```python
from build123d import *

# Parameters (mm, degrees)
SKETCH1_W           = 16
SKETCH1_H           = 16
BOSS_EXTRUDE1_DEPTH = 10
SKETCH4_R           = 1.75
CUT_EXTRUDE3_DEPTH  = 10
CUT_EXTRUDE4_DEPTH  = 7.5
FILLET1_R           = 1
FILLET2_R           = 1.75
FILLET5_R           = 3
CHAMFER1_SIZE       = 1
FILLET6_R           = 0.5
SKETCH6_R           = 2
CUT_EXTRUDE5_DEPTH  = 2


with BuildPart() as part:
    # Sketch1 → Boss-Extrude1 (new body)
    with BuildSketch(Plane(origin=(0, 0, 0), x_dir=(1, 0, 0), z_dir=(0, 1, 0))):
        with Locations((8, -8)):
            Rectangle(SKETCH1_W, SKETCH1_H)
    extrude(amount=BOSS_EXTRUDE1_DEPTH)

    # Sketch4 → Cut-Extrude3 (cut)
    with BuildSketch(Plane(origin=(0, 10, 0), x_dir=(1, 0, 0), z_dir=(0, 1, 0))):
        with Locations(Location((5, -11, 0), (0, 0, 270))):
            Circle(SKETCH4_R)
    extrude(amount=-CUT_EXTRUDE3_DEPTH, mode=Mode.SUBTRACT)

    # Sketch5 → Cut-Extrude4 (cut)
    with BuildSketch(Plane(origin=(0, 10, 0), x_dir=(1, 0, 0), z_dir=(0, 1, 0))):
        Polygon((0, -2.35), (13.65, -2.35), (13.65, -16), (10.35, -16), (10.35, -5.65), (0, -5.65), align=None)
    extrude(amount=-CUT_EXTRUDE4_DEPTH, mode=Mode.SUBTRACT)

    # Fillet1
    fillet1_edges = [part.edges().sort_by_distance(p)[0] for p in [
        (10.35, 6.25, 5.65),
    ]]
    fillet(fillet1_edges, radius=FILLET1_R)

    # Fillet2
    fillet2_edges = [part.edges().sort_by_distance(p)[0] for p in [
        (13.65, 6.25, 2.35),
    ]]
    fillet(fillet2_edges, radius=FILLET2_R)

    # Fillet5
    fillet5_edges = [part.edges().sort_by_distance(p)[0] for p in [
        (16, 5, 0),
    ]]
    fillet(fillet5_edges, radius=FILLET5_R)

    # Chamfer1
    chamfer1_edges = [part.edges().sort_by_distance(p)[0] for p in [
        (0, 6.25, 5.65),
        (0, 6.25, 2.35),
        (13.65, 6.25, 16),
        (10.35, 6.25, 16),
    ]]
    chamfer(chamfer1_edges, length=CHAMFER1_SIZE)

    # Fillet6
    fillet6_edges = [part.edges().sort_by_distance(p)[0] for p in [
        (0, 5, 0),
        (16, 5, 16),
        (0, 5, 16),
    ]]
    fillet(fillet6_edges, radius=FILLET6_R)

    # Sketch6 → Cut-Extrude5 (cut)
    with BuildSketch(Plane(origin=(0, 10, 0), x_dir=(1, 0, 0), z_dir=(0, 1, 0))):
        with Locations(Location((5, -11, 0), (0, 0, 270))):
            Circle(SKETCH6_R)
    extrude(amount=-CUT_EXTRUDE5_DEPTH, mode=Mode.SUBTRACT)


solid = part.part
```
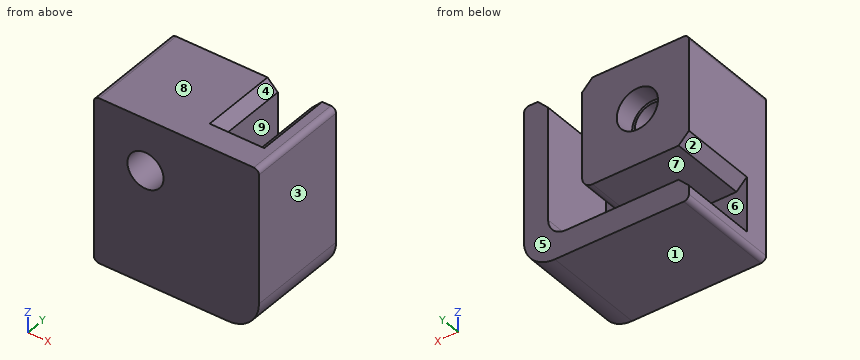
Check sheet for the modelled part. Datum: model origin and axes. Units: mm. Face numbers are marked on the shaded views. A direction names the side the tool comes from. Round coordinates to 2 decimals unless told otherwise and drop trailing zeros. Loops run counter-clockwise (first coordinate to the right, second up) from the corner with the lowest first, then second, coordinate; pieces in that order, holes last. Notation, with made-up numbers: (-5, 42.25) - (52, 42.25) arc R26 ccw to (52, 69.25) - close; hole circle Ø1 at (-15.5, -37.5). An arc over 180 degrees is marked (long way). Answer as a JSON object with one key per item and string values. Group by question number.
Q1. Sectioned sample at A-A, the plane z = 11. Enter the section's corners in (x, y).
Q2. Sectioned sample at D-D, the plane z = 14.5. Enter the section's corners in (x, y), plus the area to 3 significant figures.
Q3. Sectioned sample at B-B, the plane y = 7.5. Enter the section's corners in (x, z).
Q4. Scan lines: line 1 along X through (y, z) = (9.6, 11); line 2 along X through (y, z) = (6.25, 11); line 3 along Z through (x, y) = (1.5, 8). Record each from-to range of solid material in increasing order. Write a range as [from, to].
Q5. Mould release check, pull along Z, two halves, no side actions. Record for the marked faces 1, 2, 3 and 4: released by +Z, released by -Z, zero draft, split by the parting line, or undercut.
Q6. Sectioned sample at C-C, the plane x = 5. Enter the section's corners in (y, z), plus the area to 4 significant figures.
Q7. Set-up check for the marked faces 5, 6, 7, 8 and 9: record each of +Z, -Z, +X, -X, +Y, -Y from which the full face is reachable in a straight line by a thin tool's end or side.
Solution:
{
 "1": {"outline": "(0, 0) - (3.25, 0) - (3.25, 8) - (3, 8) - (3, 10) - (0, 10) - close; (6.75, 0) - (16, 0) - (16, 10) - (13.65, 10) - (13.65, 2.5) - (10.35, 2.5) - (10.35, 10) - (7, 10) - (7, 8) - (6.75, 8) - close"},
 "2": {"outline": "(0, 0) - (16, 0) - (16, 10) - (13.65, 10) - (13.65, 2.5) - (10.35, 2.5) - (10.35, 10) - (0, 10) - close", "area": "135 mm²"},
 "3": {"outline": "(0, 0.5) arc R0.5 ccw to (0.5, 0) - (13, 0) arc R3 ccw to (16, 3) - (16, 15.5) arc R0.5 ccw to (15.5, 16) - (14.65, 16) - (13.65, 15) - (13.65, 4.1) arc R1.75 cw to (11.9, 2.35) - (1, 2.35) - (0, 1.35) - close; (0, 6.65) - (1, 5.65) - (9.35, 5.65) arc R1 ccw to (10.35, 6.65) - (10.35, 15) - (9.35, 16) - (0.5, 16) arc R0.5 ccw to (0, 15.5) - close; hole circle Ø3.5 at (5, 11)"},
 "4": {"line 1": "x = [0, 3], [7, 10.35], [13.65, 16]", "line 2": "x = [0, 3.25], [6.75, 10.35], [13.65, 16]", "line 3": "z = [0, 2.35], [5.65, 16]"},
 "5": {"face 1": "released by -Z", "face 2": "undercut", "face 3": "zero draft", "face 4": "released by +Z"},
 "6": {"outline": "(0, 0) - (10, 0) - (10, 2.35) - (2.5, 2.35) - (2.5, 5.65) - (10, 5.65) - (10, 9) - (8, 9) - (8, 9.25) - (0, 9.25) - close; (0, 12.75) - (8, 12.75) - (8, 13) - (10, 13) - (10, 16) - (0, 16) - close", "area": "99.25 mm²"},
 "7": {"face 5": "+Z, -Z, +X, -X, +Y", "face 6": "+Y", "face 7": "-X, +Y", "face 8": "+Z, +X, -X, +Y, -Y", "face 9": "+Z, +Y"}
}
